```python
from build123d import *

# Parameters (mm, degrees)
SKETCH1_W           = 6.604
SKETCH1_H           = 2.667
BOSS_EXTRUDE1_DEPTH = 6.35


with BuildPart() as part:
    # Sketch1 → Boss-Extrude1 (new body)
    with BuildSketch(Plane(origin=(0, 0, 0), x_dir=(1, 0, 0), z_dir=(0, 1, 0))):
        Polygon((54.99261314, 31.75), (0, 63.5), (-54.99261314, 31.75), (-54.99261314, -31.75), (0, -63.5), (54.99261314, -31.75), align=None)
        Polygon((-42.961556491, 33.768423119), (-39.659556491, 28.049191352), (-37.349866739, 29.382691352), (-40.651866739, 35.101923119), align=None, mode=Mode.SUBTRACT)
        with Locations((-47.423090512, 18.988087748)):
            Rectangle(SKETCH1_W, SKETCH1_H, mode=Mode.SUBTRACT)
        Polygon((-10.073223773, 52.756510867), (-7.763534021, 54.090010867), (-4.461534021, 48.3707791), (-6.771223773, 47.0372791), align=None, mode=Mode.SUBTRACT)
        Polygon((7.763534021, 54.090010867), (4.461534021, 48.3707791), (6.771223773, 47.0372791), (10.073223773, 52.756510867), align=None, mode=Mode.SUBTRACT)
        Polygon((40.651866739, 35.101923119), (42.961556491, 33.768423119), (39.659556491, 28.049191352), (37.349866739, 29.382691352), align=None, mode=Mode.SUBTRACT)
        with Locations((47.423090512, 18.988087748)):
            Rectangle(SKETCH1_W, SKETCH1_H, mode=Mode.SUBTRACT)
        with Locations((47.423090512, -18.988087748)):
            Rectangle(SKETCH1_W, SKETCH1_H, mode=Mode.SUBTRACT)
        Polygon((42.961556491, -33.768423119), (39.659556491, -28.049191352), (37.349866739, -29.382691352), (40.651866739, -35.101923119), align=None, mode=Mode.SUBTRACT)
        Polygon((10.073223773, -52.756510867), (7.763534021, -54.090010867), (4.461534021, -48.3707791), (6.771223773, -47.0372791), align=None, mode=Mode.SUBTRACT)
        Polygon((-7.763534021, -54.090010867), (-4.461534021, -48.3707791), (-6.771223773, -47.0372791), (-10.073223773, -52.756510867), align=None, mode=Mode.SUBTRACT)
        Polygon((-40.651866739, -35.101923119), (-42.961556491, -33.768423119), (-39.659556491, -28.049191352), (-37.349866739, -29.382691352), align=None, mode=Mode.SUBTRACT)
        with Locations((-47.423090512, -18.988087748)):
            Rectangle(SKETCH1_W, SKETCH1_H, mode=Mode.SUBTRACT)
    extrude(amount=BOSS_EXTRUDE1_DEPTH)


solid = part.part
```
Can you work these out from the model? Positions are in its coordinate system, mm. A direction names the side the tool comes from. Coordinates: 2 decimals unless noted, no trailing zeros. Loops run counter-clockwise (first coordinate to the right, second up) from the corner with the lowest first, then second, coordinate; pieces in that order, holes last. Notation, with made-up numbers: (-19, -20.75) -> (-1, -20.75) arc R14 cw to (-1, -11.75) -> close; hole circle Ø3 at (47, 52.25). An arc over 180 degrees is marked (long way). Put each result on its own line as item: value. Start each with the question number.
Q1. I want a section at A-A (x = 48). Write out the boundary of the cut face in (y, z), plus the area to 3 significant figures.
Q2. I want a section at C-C (z = -38). Write out the boundary of the cut face in (x, y), plus the area to 3 significant figures.
Q3. I want a section at D-D (x = -31). Write out the boundary of the cut face in (y, z).
Q4. If I drill on line 1 (Z direction, x = -8, y = 5); line 2 (X direction, y = 3, z = 33); line 3 (Z direction, x = -6, y = 5.75), over which ranges is the centre line in solid material (lowest first)? Write a range as [from, to].
Q5. Thinking about a two-plate mould opening in X: for faces 3 (the face through (47, 3, 20.322)), 4 (the face through (27.881, 3.131, -47.403)), 5 (the face through (-54.993, 3, 0)), which applies, pulls with the +X half, pulls with the -X half, needs draft (parallel to the pull), parting line crosses it, or undercut?
Q6. I want a section at B-B (y = 1.5). Count the separate pieces of the cut face and the enclosed holes in it, plus the area to 3 significant figures.
Q7. I'm going to push flat-ended pins straight in: P1, Ø1, axis at x = 35.5, y = 2.5, coming from the +Z side; P2, Ø3, axis at x = 47, y = 1.5, coming from the +Z side; P3, Ø3, axis at x = 47.5, y = 4.5, coming from the -Z side. Where does each tip first touch, or does it pass through?
Q8. For faces 1 (the face through (-27.881, 3.131, 47.403)), 2 (the face through (-8.4, 3.13, -49.86)), which set-ups out of +Z, -Z, +X, -X, +Y, -Y let a thin tool reach every point of the face, with its end or its side?
Taken from the geometry:
1. outline: (0, -35.79) -> (6.35, -35.79) -> (6.35, -20.32) -> (0, -20.32) -> close; (0, -17.65) -> (6.35, -17.65) -> (6.35, 17.65) -> (0, 17.65) -> close; (0, 20.32) -> (6.35, 20.32) -> (6.35, 35.79) -> (0, 35.79) -> close
1. area: 421 mm2
2. outline: (-44.17, 0) -> (44.17, 0) -> (44.17, 6.35) -> (-44.17, 6.35) -> close
2. area: 561 mm2
3. outline: (0, -45.6) -> (6.35, -45.6) -> (6.35, 45.6) -> (0, 45.6) -> close
4. line 1: z = [-58.88, -53.95], [-49.17, 49.17], [53.95, 58.88]
4. line 2: x = [-52.83, -42.52], [-39.44, 39.44], [42.52, 52.83]
4. line 3: z = [-60.04, -51.04], [-47.48, 47.48], [51.04, 60.04]
5. face 3: undercut
5. face 4: pulls with the +X half
5. face 5: pulls with the -X half
6. separate pieces: 1
6. enclosed holes: 12
6. area: 10,300 mm2
7. P1: stops at z = 43.29
7. P2: stops at z = 37.23
7. P3: stops at z = -36.94
8. face 1: +Z, -X, +Y, -Y
8. face 2: +Y, -Y
